For this review, use the dimensioned drawing (mm, ordinates from the lowest corner) and the shaded views. A direction names the side the tool comes from. Coordinates: 2 decimals unless noted, no trailing zeros. Loops run counter-clockwise (first coordinate to the right, second up) from the corner with the lowest first, then second, coordinate; pieces in that order, holes last. Notation, with made-up numbers: (10, -4) - (16, -4) arc R5 cw to (16, 3) - close; hole circle Ø7 at (20.25, 0.25). An arc over 180 degrees is marked (long way). Answer in a Markdown table with one row per item. Add a question column.
(1) We need section D-D, the plane x = 15. Write out the cut boundary in (y, z), plus the area to 3 significant figures.
(2) The part is to be moulded in two halves that separate along X. For the marked faces 1, 2 and 3, say which applies: released by +X, released by -X, zero draft, split by the parting line, or undercut.
(3) To check wall thickness, follow L1, parallel to X at y = 11.5, z = 30; L2, parallel to X at y = 2.5, z = 10; L3, parallel to Z at x = 15, y = 12.3. State the ranges of each line that lie inside material, in increasing order. Write a range as [from, to].
(4) We need section C-C, the plane z = 15. Write out the cut boundary in (x, y), plus the area to 3 significant figures.
(5) We need section B-B, the plane x = 75. Write out the cut boundary in (y, z).
(6) Clearance check with flat-ended pins moving along their axes: pin 1 (1.4 mm diameter, centred on x = 64.5, z = 10.5, fed in from +Y); pin 2 (1 mm diameter, centred on y = 6, z = 34, fed in from +X); pin 3 (1 mm diameter, centred on x = 50, y = 12, fed in from -Z); pin 4 (2.5 mm diameter, centred on x = 75, z = 10, fed in from +Y). State where each tip first meets the part, or that it passes through.
(7) We need section A-A, the plane z = 10. Write out the cut boundary in (x, y), plus the area to 3 significant figures.
(8) For the marked faces 4, 5, 6, 7 and 8, list the 3-axis set-ups (+Z, -Z, +X, -X, +Y, -Y) from which the entire face can be reached by the end or side of a thin tool; tool diameter is ignored.
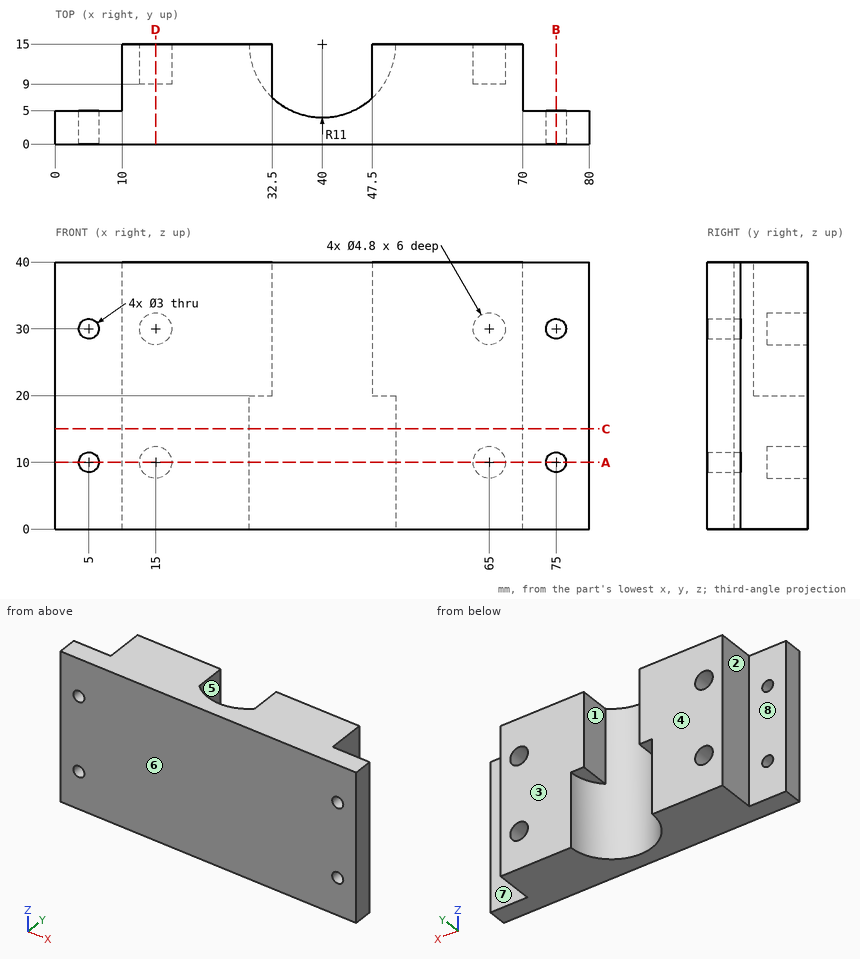
Responses:
| question | item | result |
|---|---|---|
| 1 | outline | (0, 0) - (15, 0) - (15, 7.6) - (9, 7.6) - (9, 12.4) - (15, 12.4) - (15, 27.6) - (9, 27.6) - (9, 32.4) - (15, 32.4) - (15, 40) - (0, 40) - close |
| 1 | area | 542 mm2 |
| 2 | face 1 | undercut |
| 2 | face 2 | released by -X |
| 2 | face 3 | zero draft |
| 3 | L1 | x = [10, 12.6], [17.4, 32.5], [47.5, 62.6], [67.4, 70] |
| 3 | L2 | x = [0, 3.5], [6.5, 73.5], [76.5, 80] |
| 3 | L3 | z = [0, 7.6], [12.4, 27.6], [32.4, 40] |
| 4 | outline | (0, 0) - (80, 0) - (80, 5) - (70, 5) - (70, 15) - (51, 15) arc R11 cw to (29, 15) - (10, 15) - (10, 5) - (0, 5) - close |
| 4 | area | 810 mm2 |
| 5 | outline | (0, 0) - (5, 0) - (5, 8.5) - (0, 8.5) - close; (0, 11.5) - (5, 11.5) - (5, 28.5) - (0, 28.5) - close; (0, 31.5) - (5, 31.5) - (5, 40) - (0, 40) - close |
| 6 | pin 1 | stops at y = 9 |
| 6 | pin 2 | stops at x = 70 |
| 6 | pin 3 | stops at z = 20 |
| 6 | pin 4 | passes through |
| 7 | outline | (0, 0) - (3.5, 0) - (3.5, 5) - (0, 5) - close; (6.5, 0) - (73.5, 0) - (73.5, 5) - (70, 5) - (70, 15) - (67.4, 15) - (67.4, 9) - (62.6, 9) - (62.6, 15) - (51, 15) arc R11 cw to (29, 15) - (17.4, 15) - (17.4, 9) - (12.6, 9) - (12.6, 15) - (10, 15) - (10, 5) - (6.5, 5) - close; (76.5, 0) - (80, 0) - (80, 5) - (76.5, 5) - close |
| 7 | area | 722 mm2 |
| 8 | face 4 | +Z, -Z, +X, -X, +Y |
| 8 | face 5 | +Z, -Z, +Y |
| 8 | face 6 | +Z, -Z, +X, -X, -Y |
| 8 | face 7 | +Z, -Z, +X, +Y |
| 8 | face 8 | +Z, -Z, -X, +Y |
